Could you check a few things on this model? Use its own coordinates, in mm. A direction names the side the tool comes from. Coordinates: 2 decimals unless noted, no trailing zeros. Loops run counter-clockwise (first coordinate to the right, second up) from the corner with the lowest first, then second, coordinate; pieces in that order, holes last.
from build123d import *

# Parameters (mm, degrees)
SKETCH1_R           = 1.778
BOSS_EXTRUDE1_DEPTH = 6.5
CUT_EXTRUDE1_DEPTH  = 4
CHAMFER1_SIZE       = 1.905
CHAMFER1_SIZE2      = 3.81


with BuildPart() as part:
    # Sketch1 → Boss-Extrude1 (new body)
    with BuildSketch(Plane(origin=(0, 0, 0), x_dir=(1, 0, 0), z_dir=(0, 1, 0))):
        with BuildLine():
            Line((14.722227154, 13.97), (29.21, 13.97))
            ThreePointArc((29.21, 13.97), (33.700128061, 12.110128061), (35.56, 7.62))
            Line((35.56, 7.62), (35.56, -7.62))
            ThreePointArc((35.56, -7.62), (33.700128061, -12.110128061), (29.21, -13.97))
            Line((29.21, -13.97), (19.176579466, -13.97))
            ThreePointArc((19.176579466, -13.97), (16.831686562, -14.418815604), (14.818265951, -15.701818182))
            ThreePointArc((14.818265951, -15.701818182), (0, -21.59), (-14.818265951, -15.701818182))
            ThreePointArc((-14.818265951, -15.701818182), (-16.831686562, -14.418815604), (-19.176579466, -13.97))
            Line((-19.176579466, -13.97), (-29.21, -13.97))
            ThreePointArc((-29.21, -13.97), (-33.700128061, -12.110128061), (-35.56, -7.62))
            Line((-35.56, -7.62), (-35.56, 7.62))
            ThreePointArc((-35.56, 7.62), (-33.700128061, 12.110128061), (-29.21, 13.97))
            Line((-29.21, 13.97), (-14.722227154, 13.97))
            ThreePointArc((-14.722227154, 13.97), (-13.078726217, 13.753628997), (-11.547227154, 13.119261314))
            Line((-11.547227154, 13.119261314), (-8.995011096, 11.645738686))
            ThreePointArc((-8.995011096, 11.645738686), (-7.463512032, 11.011371003), (-5.820011096, 10.795))
            Line((-5.820011096, 10.795), (5.820011096, 10.795))
            ThreePointArc((5.820011096, 10.795), (7.463512032, 11.011371003), (8.995011096, 11.645738686))
            Line((8.995011096, 11.645738686), (11.547227154, 13.119261314))
            ThreePointArc((11.547227154, 13.119261314), (13.078726217, 13.753628997), (14.722227154, 13.97))
        make_face()
        with Locations(Location((0, 0, 0), (0, 0, 270))):  # turned: the seam where the file's is
            Circle(SKETCH1_R, mode=Mode.SUBTRACT)
        with BuildLine():
            Line((-23.495, -2.667), (-29.21, -2.667))
            ThreePointArc((-29.21, -2.667), (-31.877, 0), (-29.21, 2.667))
            Line((-29.21, 2.667), (-23.495, 2.667))
            ThreePointArc((-23.495, 2.667), (-20.828, 0), (-23.495, -2.667))
        make_face(mode=Mode.SUBTRACT)
        with BuildLine():
            Line((23.495, 2.667), (29.21, 2.667))
            ThreePointArc((29.21, 2.667), (31.877, 0), (29.21, -2.667))
            Line((29.21, -2.667), (23.495, -2.667))
            ThreePointArc((23.495, -2.667), (20.828, 0), (23.495, 2.667))
        make_face(mode=Mode.SUBTRACT)
        with BuildLine():
            Line((-15.289419162, 6.517949192), (-13.089714637, 5.247949192))
            ThreePointArc((-13.089714637, 5.247949192), (-10.357663829, 5.98), (-11.089714637, 8.712050808))
            Line((-11.089714637, 8.712050808), (-13.289419162, 9.982050808))
            ThreePointArc((-13.289419162, 9.982050808), (-16.02146997, 9.25), (-15.289419162, 6.517949192))
        make_face(mode=Mode.SUBTRACT)
        with BuildLine():
            Line((13.289419162, 9.982050808), (11.089714637, 8.712050808))
            ThreePointArc((11.089714637, 8.712050808), (10.357663829, 5.98), (13.089714637, 5.247949192))
            Line((13.089714637, 5.247949192), (15.289419162, 6.517949192))
            ThreePointArc((15.289419162, 6.517949192), (16.02146997, 9.25), (13.289419162, 9.982050808))
        make_face(mode=Mode.SUBTRACT)
        with BuildLine():
            Line((2, -16.5), (2, -13.96))
            ThreePointArc((2, -13.96), (0, -11.96), (-2, -13.96))
            Line((-2, -13.96), (-2, -16.5))
            ThreePointArc((-2, -16.5), (0, -18.5), (2, -16.5))
        make_face(mode=Mode.SUBTRACT)
    extrude(amount=BOSS_EXTRUDE1_DEPTH)

    # Sketch5 → Cut-Extrude1 (cut)
    with BuildSketch(Plane(origin=(0, 6.5, 0), x_dir=(1, 0, 0), z_dir=(0, 1, 0))):
        with BuildLine():
            Line((-3.96875, -13.96), (-3.96875, -16.5))
            ThreePointArc((-3.96875, -16.5), (0, -20.46875), (3.96875, -16.5))
            Line((3.96875, -16.5), (3.96875, -13.96))
            ThreePointArc((3.96875, -13.96), (0, -9.99125), (-3.96875, -13.96))
        make_face()
        with BuildLine():
            Line((12.305044162, 11.687038321), (10.105339637, 10.417038321))
            ThreePointArc((10.105339637, 10.417038321), (8.652676316, 4.995625), (14.074089637, 3.542961679))
            Line((14.074089637, 3.542961679), (16.273794162, 4.812961679))
            ThreePointArc((16.273794162, 4.812961679), (17.726457484, 10.234375), (12.305044162, 11.687038321))
        make_face()
        with BuildLine():
            Line((-12.305044162, 11.687038321), (-10.105339637, 10.417038321))
            ThreePointArc((-10.105339637, 10.417038321), (-8.652676316, 4.995625), (-14.074089637, 3.542961679))
            Line((-14.074089637, 3.542961679), (-16.273794162, 4.812961679))
            ThreePointArc((-16.273794162, 4.812961679), (-17.726457484, 10.234375), (-12.305044162, 11.687038321))
        make_face()
    extrude(amount=-CUT_EXTRUDE1_DEPTH, mode=Mode.SUBTRACT)

    # Chamfer1
    chamfer1_edges = [part.edges().sort_by_distance(p)[0] for p in [
        (0, 6.5, -1.778),
    ]]
    chamfer1_side = [part.faces().sort_by_distance(p)[0] for p in [
        (0, 6.5, 2.195443335),
    ]]
    chamfer(chamfer1_edges, length=CHAMFER1_SIZE, length2=CHAMFER1_SIZE2, reference=chamfer1_side[0])


solid = part.part
1) Imagine slicing it at C-C on y = 1.5. State how many separate pieces and enclosed holes the cut face has, plus the area to 3 significant figures.
2) Will these pins go through, and if not, where does the flat tip stop? pin 1 (1.3 mm diameter, centred on y = 4, z = 15.5, fed in from +X); pin 2 (2 mm diameter, centred on y = 4, z = 16, fed in from -X); pin 3 (1 mm diameter, centred on y = 3, z = 18, fed in from +X).
3) Imagine slicing it at B-B on x = -30.5. List the corners of the cut face in (y, z) for me.
4) We'd pull the mould along Z, two halves only. Please class faces 5 (the cylindrical face through (-10.38, 1.23, -5.94)), 6 (the flat face through (0, 3, -10.795)), 7 (the flat face through (24, 3, 13.97)), 8 (the flat face through (-11.22, 4.53, -11.06)): released by +Z, released by -Z, zero draft, split by the parting line, or undercut.
5) If I drill on L1, parallel to X at y = 1.4, z = 0; L2, parallel to X at y = 6.25, z = -8; L3, parallel to Z at x = -25.5, y = 4, over which ranges is the centre line in solid material (lowest first)?
6) For faces 1 (the flat face through (0, 6.5, 8)), 2 (the cylindrical face through (7.441, 3.204, -11.005)), 3 (the flat face through (-12, 2.5, -10)), 4 (the cylindrical face through (0.04, 1.23, 11.96)), which set-ups out of +Z, -Z, +X, -X, +Y, -Y let a thin tool reach every point of the face, with its end or its side?
7) Imagine slicing it at A-A on x = 0. List the corners of the cut face in (y, z) for me (3 decimals).
Solved:
1. separate pieces: 1
1. enclosed holes: 6
1. area: 1,880 mm2
2. pin 1: stops at x = 15.95
2. pin 2: stops at x = -15.71
2. pin 3: stops at x = 12.64
3. outline: (0, -13.84) - (6.5, -13.84) - (6.5, -2.33) - (0, -2.33) - close; (0, 2.33) - (6.5, 2.33) - (6.5, 13.84) - (0, 13.84) - close
4. face 5: undercut
4. face 6: released by -Z
4. face 7: released by +Z
4. face 8: undercut
5. L1: x = -35.56 to -31.88, -20.83 to -1.78, 1.78 to 20.83, 31.88 to 35.56
5. L2: x = -35.55 to -18.25, -8.25 to 8.25, 18.25 to 35.55
5. L3: z = -13.97 to -2.67, 2.67 to 13.97
6. face 1: +Z, -Z, +X, -X, +Y
6. face 2: -Z, +Y, -Y
6. face 3: +Y
6. face 4: +Y, -Y
7. outline: (0, -10.795) - (6.5, -10.795) - (6.5, -3.683) - (2.69, -1.778) - (0, -1.778) - close; (0, 1.778) - (2.69, 1.778) - (6.5, 3.683) - (6.5, 9.991) - (2.5, 9.991) - (2.5, 11.96) - (0, 11.96) - close; (0, 18.5) - (2.5, 18.5) - (2.5, 20.469) - (6.5, 20.469) - (6.5, 21.59) - (0, 21.59) - close
